Here's how the part is built. I have some questions about the finished solid (model axes, mm). Face numbers are marked on the shaded views. A direction names the side the tool comes from. Round coordinates to 2 decimals unless told otherwise and drop trailing zeros. Loops run counter-clockwise (first coordinate to the right, second up) from the corner with the lowest first, then second, coordinate; pieces in that order, holes last. Notation, with made-up numbers: M 78.5,68 L 130.5,68 A9 ccw 130.5,77 Z; hole C 79,73.25 d11. An arc over 180 degrees is marked long. Write each question's results on one line, items separated by ' | '. Start each with the question number.
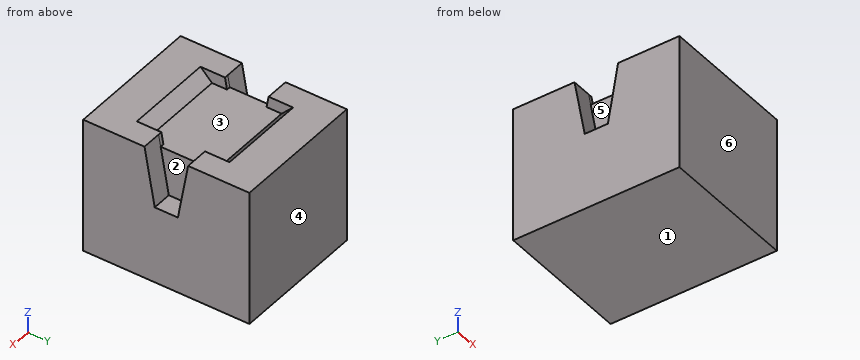
```python
from build123d import *

# Parameters (mm, degrees)
EXTRUDE002_DEPTH = 5
SKETCH003_W      = 125
SKETCH003_H      = 90
EXTRUDE001_DEPTH = 70
SKETCH002_W      = 125
SKETCH002_H      = 120
EXTRUDE_DEPTH    = 176


with BuildPart() as extrude002:
    # Sketch004 (on Face1 of Extrude001) → Extrude002 (new body)
    with BuildSketch(Plane(origin=(25.5, 0, 0), x_dir=(0, -1, 0), z_dir=(-1, 0, 0))):
        Polygon((-81.970381, 160), (-62.55, 160), (-47.55, 175), (-79.325476, 175), align=None)
        Polygon((-133.129619, 160), (-135.774524, 175), (-167.55, 175), (-152.55, 160), align=None)
    extrude(amount=-EXTRUDE002_DEPTH)


with BuildPart() as extrude002_mirrored:
    # Mirror: instance of Extrude002
    add(extrude002.part.mirror(Plane(origin=(88, 0, 0), x_dir=(0, -1, 0), z_dir=(1, 0, 0))))


with BuildPart() as extrude001:
    # Sketch003 → Extrude001 (new body)
    with BuildSketch(Plane.XY.offset(160)):
        with Locations((88, 107.55)):
            Rectangle(SKETCH003_W, SKETCH003_H)
    extrude(amount=-EXTRUDE001_DEPTH)


with BuildPart() as loft_body:
    # Sketch002 (on Face1 of Extrude) → Loft section 0
    with BuildSketch(Plane.XY.offset(175)):
        with Locations((88, 107.55)):
            Rectangle(SKETCH002_W, SKETCH002_H)
    # Sketch003 → Loft section 1
    with BuildSketch(Plane.XY.offset(160)):
        with Locations((88, 107.55)):
            Rectangle(SKETCH003_W, SKETCH003_H)
    loft(ruled=True)


with BuildPart() as fusion001:
    # Sketch001 → Extrude (new body)
    with BuildSketch(Plane.YZ):
        Polygon((0, 0), (215.1, 0), (215.1, 175), (135.774524, 175), (122.55, 100), (92.55, 100), (79.325476, 175), (0, 175), align=None)
    extrude(amount=EXTRUDE_DEPTH)

    # Cut: cut Loft body
    add(loft_body.part, mode=Mode.SUBTRACT)

    # Fusion: union Extrude001
    add(extrude001.part)

    # Fusion001: union Extrude002 (mirrored), Extrude002
    add(extrude002_mirrored.part)
    add(extrude002.part)


solid = fusion001.part
```
1. I want a section at A-A on x = 85. List the corners of the cut face in (y, z) for me, plus the area to 3 significant figures.
2. I want a section at B-B on y = 156. List the corners of the cut face in (x, z) for me, plus the area to 3 significant figures.
3. If we mould it in two halves opening along Y, with no side actions, what happens to the marked faces 4, 5 and 6? For each: released by +Y, released by -Y, zero draft, split by the parting line, or undercut.
4. For pin 1 (15.5 mm diameter, centred on y = 108.5, z = 128, fed in from -X); pin 2 (13 mm diameter, centred on x = 159.5, y = 104, fed in from +Z); pin 3 (6 mm diameter, centred on x = 26.5, y = 99.5, fed in from +Z), each with a flat end and sliding along its axis, tell me the tip position at first contact or that it passes through.
5. I want a section at C-C on z = 109. List the corners of the cut face in (x, y) for me.
6. Which directions (+Z, -Z, +X, -X, +Y, -Y) give clear straight access to the entire face, cutting with the end or side of a thin tool? Please do the marked faces 1, 2 and 3.
7. I need wall thicknesses on line 1 along Z through (x, y) = (137, 83); line 2 along Y through (x, z) = (160.5, 110.5); line 3 along Y through (x, z) = (11, 152.5). Which ranges of each line are inside material? Lowest first, please.
Outcome:
1) outline: M 0,0 L 215.1,0 L 215.1,175 L 167.55,175 L 152.55,160 L 62.55,160 L 47.55,175 L 0,175 Z | area: 36,100 mm2
2) outline: M 0,0 L 176,0 L 176,175 L 145.5,175 L 145.5,163.45 L 30.5,163.45 L 30.5,175 L 0,175 Z | area: 29,500 mm2
3) face 4: released by +Y | face 5: undercut | face 6: released by -Y
4) pin 1: x = 25.5 | pin 2: z = 100 | pin 3: z = 160
5) outline: M 0,0 L 176,0 L 176,90.96 L 150.5,90.96 L 150.5,124.14 L 176,124.14 L 176,215.1 L 0,215.1 L 0,124.14 L 25.5,124.14 L 25.5,90.96 L 0,90.96 Z
6) face 1: -Z, +X, -X, +Y, -Y | face 2: +Z, +X | face 3: +Z
7) line 1: 0 to 160 | line 2: 0 to 90.7, 124.4 to 215.1 | line 3: 0 to 83.29, 131.81 to 215.1
